```python
from build123d import *

# Parameters (mm, degrees)
SKETCH1_W                               = 70
SKETCH1_H                               = 50
BOSS_EXTRUDE1_DEPTH                     = 48
CBORE_FOR_M8_HEX_HEAD_BOLT1_D           = 8.6
CBORE_FOR_M8_HEX_HEAD_BOLT1_CBORE_D     = 14
CBORE_FOR_M8_HEX_HEAD_BOLT1_CBORE_DEPTH = 11
M25_CLEARANCE_HOLE1_D                   = 28.4
F_4_2_4_2_DIAMETER_HOLE1_D              = 4.2
F_4_2_4_2_DIAMETER_HOLE1_DEPTH          = 14
F_4_2_4_2_DIAMETER_HOLE1_TIP            = 1.2618073
SKETCH8_W                               = 70
SKETCH8_H                               = 7
CUT_EXTRUDE1_DEPTH                      = 66.582009728
CHAMFER1_SIZE                           = 3


with BuildPart() as part:
    # Sketch1 → Boss-Extrude1 (new body)
    with BuildSketch(Plane.XZ.offset(24)):
        Rectangle(SKETCH1_W, SKETCH1_H)
    extrude(amount=-BOSS_EXTRUDE1_DEPTH)

    # CBORE for M8 Hex Head Bolt1 (through all)
    with Locations(Plane(origin=(0, -24, 0), x_dir=(-1, 0, 0), z_dir=(0, -1, 0))):
        with Locations((25, -5), (-25, -5), (-25, 15), (25, 15)):
            CounterBoreHole(CBORE_FOR_M8_HEX_HEAD_BOLT1_D / 2, CBORE_FOR_M8_HEX_HEAD_BOLT1_CBORE_D / 2, CBORE_FOR_M8_HEX_HEAD_BOLT1_CBORE_DEPTH)

    # M25 Clearance Hole1 (through all)
    with Locations(Plane(origin=(0, 0, -25), x_dir=(-1, 0, 0), z_dir=(0, 0, -1))):
        with Locations((0, 0)):
            Hole(M25_CLEARANCE_HOLE1_D / 2)

    # Ø4.2 (4.2) Diameter Hole1
    with Locations(Plane.XY.offset(25)):
        with Locations((13.435028843, -13.435028843), (13.435028843, 13.435028843), (19, 0), (-13.435028843, 13.435028843), (-13.435028843, -13.435028843), (-19, 0)):
            Hole(F_4_2_4_2_DIAMETER_HOLE1_D / 2, depth=F_4_2_4_2_DIAMETER_HOLE1_DEPTH)
            with Locations((0, 0, -(F_4_2_4_2_DIAMETER_HOLE1_DEPTH + F_4_2_4_2_DIAMETER_HOLE1_TIP / 2))):  # 118° drill point
                Cone(0, F_4_2_4_2_DIAMETER_HOLE1_D / 2, F_4_2_4_2_DIAMETER_HOLE1_TIP, mode=Mode.SUBTRACT)

    # Sketch8 → Cut-Extrude1 (cut, through all)
    with BuildSketch(Plane.XY.offset(25)):
        with Locations((0, 20.5)):
            Rectangle(SKETCH8_W, SKETCH8_H)
        with Locations((0, -20.5)):
            Rectangle(SKETCH8_W, SKETCH8_H)
    extrude(amount=-CUT_EXTRUDE1_DEPTH, mode=Mode.SUBTRACT)

    # Chamfer1
    chamfer1_edges = [part.edges().sort_by_distance(p)[0] for p in [
        (-35, -17, 0),
        (35, -17, 0),
        (35, 17, 0),
        (-35, 17, 0),
    ]]
    chamfer(chamfer1_edges, length=CHAMFER1_SIZE - 0.0001)  # a hair under: the kernel refuses the full size


solid = part.part
```
The listing builds one solid part. Answer for the finished solid, in the listing's coordinates (mm). A direction names the side the tool comes from. Coordinates: 2 decimals unless noted, no trailing zeros. Write each loop counter-clockwise with the first axis right and the second up, starting at its lowest first coordinate (ties: lowest second). Pieces come first, ordered by that corner, then holes.
Q1. Which of the six approach directions +Z, -Z, +X, -X, +Y, -Y give full straight-line access (tool end or side, diameter ignored) to faces 4 (the cylindrical face through (16.997, 0.631, 17.902)), 5 (the cylindrical face through (-22.688, 2.21, -18.626)), 6 (the cylindrical face through (26.517, -15.028, -8.166))?
Returned:
face 4: +Z
face 5: +Y, -Y
face 6: -Y
Q2. Section C-C, the plane y = -5.5 is taken. Write down the section's boundary in (x, z).
Returned:
outline: (-35, -25) - (-13.09, -25) - (-13.09, 25) - (-35, 25) - close; (13.09, -25) - (35, -25) - (35, 25) - (13.09, 25) - close; hole circle Ø8.6 at (-25, -15); hole circle Ø8.6 at (-25, 5); hole circle Ø8.6 at (25, -15); hole circle Ø8.6 at (25, 5)
Q3. Section B-B, the plane x = 0 is taken. Write down the section's boundary in (y, z).
Returned:
outline: (-17, -25) - (-14.2, -25) - (-14.2, 25) - (-17, 25) - close; (14.2, -25) - (17, -25) - (17, 25) - (14.2, 25) - close
Q4. Section A-A, the plane z = -15 is taken. Give the number of separate pieces and of enclosed holes in the cut face, then the cut area to 3 significant figures.
Returned:
separate pieces: 3
enclosed holes: 1
area: 1,100 mm2
Q5. Section D-D, the plane x = -25 is taken. Write down the section's boundary in (y, z), then the cut area to 3 significant figures.
Returned:
outline: (-17, -25) - (17, -25) - (17, -19.3) - (-13, -19.3) - (-13, -22) - (-17, -22) - close; (-17, -8) - (-13, -8) - (-13, -10.7) - (17, -10.7) - (17, 0.7) - (-13, 0.7) - (-13, -2) - (-17, -2) - close; (-17, 12) - (-13, 12) - (-13, 9.3) - (17, 9.3) - (17, 25) - (-17, 25) - close
area: 1,070 mm2
Q6. Find the intervals of material crossed by line 1 along Z through (x, y) = (-22, 12); line 2 along Z through (x, y) = (28.5, -2); line 3 along X through (y, z) = (-12.5, 6), in increasing order.
Returned:
line 1: z = -25 to -18.08, -11.92 to 1.92, 8.08 to 25
line 2: z = -25 to -17.5, -12.5 to 2.5, 7.5 to 25
line 3: x = -35 to -29.18, -20.82 to -6.74, 6.74 to 20.82, 29.18 to 35
Q7. The mould has two halves that part along X. Classify faces 1 (the cylindrical face through (-1.85, 14.08, 0.35)), 2 (the flat face through (-8, -12, -25)), 3 (the flat face through (34, -15, 0)): released by +X, released by -X, zero draft, split by the parting line, or undercut.
Returned:
face 1: undercut
face 2: zero draft
face 3: released by +X
Q8. Given P1, Ø7.5, axis at x = 25, z = -15, coming from the +Y side; P2, Ø15.5, axis at x = -25, z = 5, coming from the -Y side; P3, Ø11, axis at x = -25, z = -15, coming from the -Y side; P4, Ø4, axis at x = -13.44, y = 13.44, coming from the +Z side, each flat-ended and moving along its own axis, determine where each tip first touches the part or whether it passes through.
Returned:
P1: passes through
P2: stops at y = -17
P3: stops at y = -13
P4: stops at z = 10.94
